Could you check a few things on this drawing? It's one solid part, dimensions in mm from its lowest x, y, z. Round coordinates to 2 decimals unless told otherwise and drop trailing zeros. Write each loop counter-clockwise with the first axis right and the second up, starting at its lowest first coordinate (ties: lowest second). Pieces come first, ordered by that corner, then holes. Notation, with made-up numbers: (86.25, 39) -> (105.25, 39) arc R18 ccw to (105.25, 44) -> close; hole circle Ø8 at (72.5, 88). An arc over 180 degrees is marked (long way). Put each result on its own line as item: value. Start each with the question number.
1) If I drill on line 1 along Z through (x, y) = (28, 12.75) (1 decimal); line 2 along X through (y, z) = (11.5, 21) (1 decimal); line 3 along X through (y, z) = (11.75, 33) (1 decimal), over which ranges is the centre line in solid material (lowest first)? Write a range as [from, to].
2) I want a section at B-B, the plane y = 8.5. List the corners of the cut face in (x, z) for me (1 decimal), then the cut area to 3 significant figures.
3) Will these pins go through, and if not, where does the flat tip stop? P1, Ø2.5, axis at x = 4.55, y = 12.06, coming from the -Z side; P2, Ø10, axis at x = 14.5, y = 10, coming from the -Z side; P3, Ø2, axis at y = 1, z = 3.5, coming from the -X side; P4, Ø3.5, axis at x = 18.5, z = 3.5, coming from the +Y side.
4) I want a section at A-A, the plane x = 9.5. List the corners of the cut face in (y, z) for me (1 decimal), then the cut area to 3 significant figures.
5) I want a section at C-C, the plane x = 14. List the corners of the cut face in (y, z) for me (1 decimal).
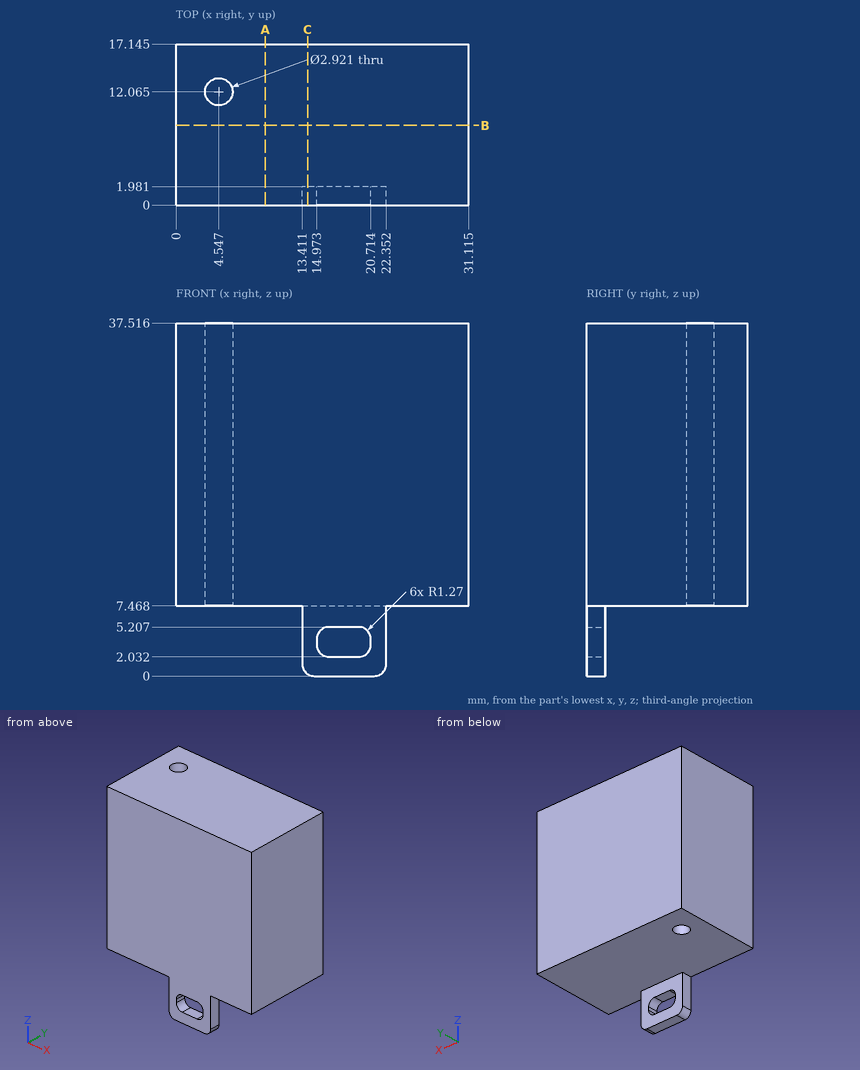
Findings:
1. line 1: z = [7.5, 37.5]
1. line 2: x = [0, 3.2], [5.9, 31.1]
1. line 3: x = [0, 3.1], [6, 31.1]
2. outline: (0, 7.5) -> (31.1, 7.5) -> (31.1, 37.5) -> (0, 37.5) -> close
2. area: 935 mm2
3. P1: passes through
3. P2: stops at z = 7.47
3. P3: stops at x = 13.41
3. P4: stops at y = 1.98
4. outline: (0, 7.5) -> (17.1, 7.5) -> (17.1, 37.5) -> (0, 37.5) -> close
4. area: 515 mm2
5. outline: (0, 0.2) -> (2, 0.2) -> (2, 7.5) -> (17.1, 7.5) -> (17.1, 37.5) -> (0, 37.5) -> close
